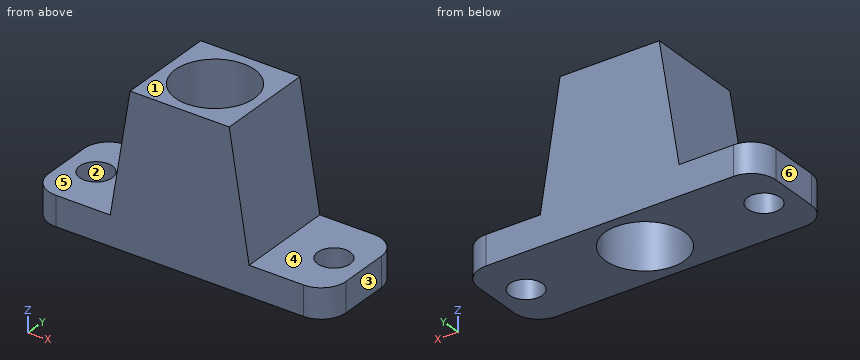
from build123d import *

# Parameters (mm, degrees)
SKETCH_1_R          = 3.3
EXTRUDE_1_DEPTH     = 6
EXTRUDE_3_DEPTH     = 20
SKETCH_3_R          = 8
CUT_EXTRUDE_1_DEPTH = 32


with BuildPart() as part:
    # 草图1 → 凸台-拉伸1 (new body)
    with BuildSketch(Plane.XY):
        with BuildLine():
            Line((25, 10), (-25, 10))
            ThreePointArc((-25, 10), (-28.535533906, 8.535533906), (-30, 5))
            Line((-30, 5), (-30, -5))
            ThreePointArc((-30, -5), (-28.535533906, -8.535533906), (-25, -10))
            Line((-25, -10), (25, -10))
            ThreePointArc((25, -10), (28.535533906, -8.535533906), (30, -5))
            Line((30, -5), (30, 5))
            ThreePointArc((30, 5), (28.535533906, 8.535533906), (25, 10))
        make_face()
        with Locations((-24, 0)):
            Circle(SKETCH_1_R, mode=Mode.SUBTRACT)
        with Locations((24, 0)):
            Circle(SKETCH_1_R, mode=Mode.SUBTRACT)
    extrude(amount=EXTRUDE_1_DEPTH)

    # 草图2 → 凸台-拉伸3 (add)
    with BuildSketch(Plane(origin=(0, 10, 0), x_dir=(1, 0, 0), z_dir=(0, 1, 0))):
        Polygon((14, -6), (-14, -6), (-10, -31), (10, -31), align=None)
    extrude(amount=-EXTRUDE_3_DEPTH)

    # 草图3 → 切除-拉伸1 (cut, through all)
    with BuildSketch(Plane.XY.offset(31)):
        Circle(SKETCH_3_R)
    extrude(amount=-CUT_EXTRUDE_1_DEPTH, mode=Mode.SUBTRACT)


solid = part.part
Read the model definition and answer for the solid it produces. Units are mm, in the model's axes. Face numbers are marked on the shaded views. A direction names the side the tool comes from. Round coordinates to 2 decimals unless told otherwise and drop trailing zeros. Write each loop counter-clockwise with the first axis right and the second up, starting at its lowest first coordinate (ties: lowest second). Pieces come first, ordered by that corner, then holes. Notation, with made-up numbers: M -11,16 L 48,16 A24 ccw 48,26 Z; hole C -33.75,3 d5. An arc over 180 degrees is marked long. Use a Markdown table: item, result.
1) Straight lines are drawn through the part: line 1 along Y through (x, z) = (24, 3.55); line 2 along Y through (x, z) = (0, 16); line 3 along X through (y, z) = (-1.5, 25.5). For each, find the intervals that lie inside material, in ascending order. Write a range as [from, to].
Answers follow:
| item | result |
|---|---|
| line 1 | y = [-10, -3.3], [3.3, 10] |
| line 2 | y = [-10, -8], [8, 10] |
| line 3 | x = [-10.88, -7.86], [7.86, 10.88] |
2) For a pull along X with two mould halves and no side action, classify the marked faces 1, 2 and 3 as pulls with the +X half, pulls with the -X half, needs draft (parallel to the pull), parting line crosses it, or undercut.
Answers follow:
| item | result |
|---|---|
| face 1 | needs draft |
| face 2 | undercut |
| face 3 | pulls with the +X half |
3) A tool of negligible diameter and unlimited length cuts with its end or side. For the marked faces 4, 5 and 6, from which of +Z, -Z, +X, -X, +Y, -Y can it reach the whole face along a straight path? Write none if from no direction.
Answers follow:
| item | result |
|---|---|
| face 4 | +Z, +X, +Y, -Y |
| face 5 | +Z, -X, +Y, -Y |
| face 6 | +Z, -Z, -X, +Y, -Y |
4) Flat-ended cylindrical pins translate along their axes: pin 1 (1.5 mm diameter, centred on y = -7, z = 7.5, fed in from +X); pin 2 (1.5 mm diameter, centred on y = -3, z = 14, fed in from +X); pin 3 (5 mm diameter, centred on x = -18.5, y = 2, fed in from +Z). Find the tip coordinate at first contact, or state that the pin passes through.
Answers follow:
| item | result |
|---|---|
| pin 1 | stops at x = 13.88 |
| pin 2 | stops at x = 12.84 |
| pin 3 | stops at z = 6 |
5) The part is cut by section D-D (y = -6). Write down the section's boundary in (x, z).
Answers follow:
| item | result |
|---|---|
| outline | M -29.9,0 L -5.29,0 L -5.29,31 L -10,31 L -14,6 L -29.9,6 Z; M 5.29,0 L 29.9,0 L 29.9,6 L 14,6 L 10,31 L 5.29,31 Z |
6) The part is cut by section A-A (y = 0). Write down the section's boundary in (x, z).
Answers follow:
| item | result |
|---|---|
| outline | M -30,0 L -27.3,0 L -27.3,6 L -30,6 Z; M -20.7,0 L -8,0 L -8,31 L -10,31 L -14,6 L -20.7,6 Z; M 8,0 L 20.7,0 L 20.7,6 L 14,6 L 10,31 L 8,31 Z; M 27.3,0 L 30,0 L 30,6 L 27.3,6 Z |
7) The part is cut by section C-C (z = 29). Write down the section's boundary in (x, y), plus the area to 3 significant figures.
Answers follow:
| item | result |
|---|---|
| outline | M -10.32,-10 L 10.32,-10 L 10.32,10 L -10.32,10 Z; hole C 0,0 d16 |
| area | 212 mm2 |
8) The part is cut by section B-B (x = -24). Write down the section's boundary in (y, z).
Answers follow:
| item | result |
|---|---|
| outline | M -10,0 L -3.3,0 L -3.3,6 L -10,6 Z; M 3.3,0 L 10,0 L 10,6 L 3.3,6 Z |
